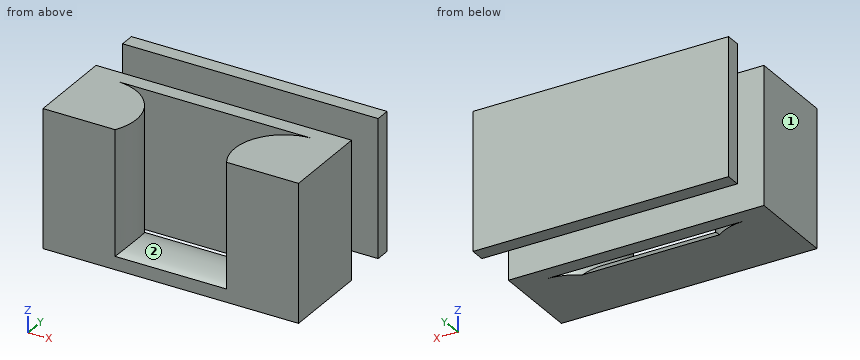
```python
from build123d import *

# Parameters (mm, degrees)
BOSS_EXTRUDE1_DEPTH = 3.5
BOSS_EXTRUDE2_DEPTH = 3.5
SKETCH4_W           = 13
SKETCH4_H           = 7
BOSS_EXTRUDE3_DEPTH = 0.75


with BuildPart() as part:
    # Sketch1 → Boss-Extrude1 (new body, symmetric)
    with BuildSketch(Plane.XY):
        with BuildLine():
            ThreePointArc((-2.834936491, -2.25), (-2.834936491, 0.25), (-5, 1.5))
            Line((-5, 1.5), (5, 1.5))
            ThreePointArc((5, 1.5), (2.834936491, 0.25), (2.834936491, -2.25))
            Line((2.834936491, -2.25), (6.5, -2.25))
            Line((6.5, -2.25), (6.5, 2.25))
            Line((6.5, 2.25), (-6.5, 2.25))
            Line((-6.5, 2.25), (-6.5, -2.25))
            Line((-6.5, -2.25), (-2.834936491, -2.25))
        make_face()
    extrude(amount=BOSS_EXTRUDE1_DEPTH, both=True)

    # Sketch2 → Boss-Extrude2 (add, symmetric)
    with BuildSketch(Plane(origin=(0, 0, 0), x_dir=(0, 0, -1), z_dir=(1, 0, 0))):
        with BuildLine():
            Line((3.5, -2.25), (3.5, 1))
            ThreePointArc((3.5, 1), (2.550755702, -0.498799074), (2.834936491, -2.25))
            Line((2.834936491, -2.25), (3.5, -2.25))
        make_face()
    extrude(amount=BOSS_EXTRUDE2_DEPTH, both=True)

    # Sketch3 → Revolve1 (revolve)
    with BuildSketch(Plane.XY):
        with BuildLine():
            Line((0, 4.5), (-1.75, 4.5))
            ThreePointArc((-1.75, 4.5), (-0.625, 3.375), (-1.75, 2.25))
            Line((-1.75, 2.25), (0, 2.25))
            Line((0, 2.25), (0, 4.5))
        make_face()
    revolve(axis=Axis((0, 5.875, 0), (0, -1, 0)))

    # Sketch4 → Boss-Extrude3 (add)
    with BuildSketch(Plane(origin=(0, 4.5, 0), x_dir=(1, 0, 0), z_dir=(0, 1, 0))):
        Rectangle(SKETCH4_W, SKETCH4_H)
    extrude(amount=BOSS_EXTRUDE3_DEPTH)


solid = part.part
```
CAD build for the part. Positions are in the model's coordinates, mm. Face numbers are marked on the shaded views. A direction names the side the tool comes from. Coordinates: 2 decimals unless noted, no trailing zeros. Loops run counter-clockwise (first coordinate to the right, second up) from the corner with the lowest first, then second, coordinate; pieces in that order, holes last. Notation, with made-up numbers: (-17, -29.5) - (41, -29.5) arc R21 ccw to (41, 6.5) - close; hole circle Ø1 at (72.5, 66.25). An arc over 180 degrees is marked (long way). Use CSV: the item, a comma, the result in double quotes. Start each with the question number.
Q1. Cut at A-A, the plane x = 5.25. List the corners of the cut face in (y, z), then the cut area to 4 significant figures.
Q2. Cut at B-B, the plane z = 2.75. List the corners of the cut face in (x, y).
Q3. Probe probe 1 along Y at (x, z) = (-3.5, -2); probe 2 along Y at (x, z) = (-5.75, 3.25); probe 3 along X at (y, z) = (-1, 2.5). List the from-to ranges inside material, lowest first. Write a range as from..to.
Q4. Cut at D-D, the plane y = 3.75. List the corners of the cut face in (x, z), then the cut area to 3 significant figures.
Q5. Cut at C-C, the plane y = 1.25. List the corners of the cut face in (x, z).
Q6. 3-axis set-ups, long thin cutter, end or side, ignore diameter. For the marked faces 1 and 2: which of +Z, -Z, +X, -X, +Y, -Y reach the whole face in a straight line?
Here are the results:
1,outline,"(-2.25, -3.5) - (2.25, -3.5) - (2.25, 3.5) - (-2.25, 3.5) - close; (4.5, -3.5) - (5.25, -3.5) - (5.25, 3.5) - (4.5, 3.5) - close"
1,area,"36.75 mm2"
2,outline,"(-6.5, -2.25) - (-2.83, -2.25) arc R2.5 ccw to (-5, 1.5) - (5, 1.5) arc R2.5 ccw to (2.83, -2.25) - (6.5, -2.25) - (6.5, 2.25) - (-6.5, 2.25) - close; (-6.5, 4.5) - (6.5, 4.5) - (6.5, 5.25) - (-6.5, 5.25) - close"
3,probe 1,"-2.25..1, 1.5..2.25, 4.5..5.25"
3,probe 2,"-2.25..2.25, 4.5..5.25"
3,probe 3,"-6.5..-2.5, 2.5..6.5"
4,outline,"circle Ø1.38 at (0, 0)"
4,area,"1.49 mm2"
5,outline,"(-6.5, -3.5) - (-3.91, -3.5) - (-3.91, 3.5) - (-6.5, 3.5) - close; (3.91, -3.5) - (6.5, -3.5) - (6.5, 3.5) - (3.91, 3.5) - close"
6,face 1,"+Z, -Z, -X, +Y, -Y"
6,face 2,"+Z"
